The listing builds one solid part. Answer for the finished solid, in the listing's coordinates (mm). A direction names the side the tool comes from. Coordinates: 2 decimals unless noted, no trailing zeros. Loops run counter-clockwise (first coordinate to the right, second up) from the corner with the lowest first, then second, coordinate; pieces in that order, holes last. Notation, with made-up numbers: M 10,-7.5 L 67,-7.5 A14 cw 67,-3.5 Z; hole C 14.25,18 d1. An arc over 180 degrees is marked long. Answer as a JSON object with one key per item and string values. Group by question number.
1. For faces 1 (the face through (5.24, 3.65, -33.55)), 2 (the face through (-14.4, -1.7, 60.5)), 3 (the face through (-21, 9, -21)), determine the directions among +Z, -Z, +X, -X, +Y, -Y from which every point of the face is accessible in a straight line to the end or side of a thin tool.
2. Straight lines are drawn through the part: L1, parallel to Y at x = 24.5, z = -32.25; L2, parallel to Z at x = 25, y = -3; L3, parallel to Y at x = -28, z = 32. For each, find the intervals that lie inside material, in ascending order.
3. Given pin 1 (2 mm diameter, centred on x = 2, y = 1, fed in from -Z); pin 2 (2.5 mm diameter, centred on x = 24.5, y = 13.5, fed in from +Z); pin 3 (1 mm diameter, centred on x = -20.5, z = -25, fed in from +Y); pin 4 (8 mm diameter, centred on x = -1, y = 4.5, fed in from +Z), each flat-ended and moving along its own axis, determine where each tip first touches the part or whether it passes through.
4. A cutting plane is placed at B-B on x = -23.5. Give the vertices of the cut face in (y, z), and give its area (3 significant figures).
5. Determine the mould class of faces 4 (the face through (32.17, 9.19, 56.11)), 5 (the face through (29.076, 6.007, 58.084)), 6 (the face through (-22.434, -0.308, 48.794)) for opening direction Y: released by +Y, released by -Y, zero draft, split by the parting line, or undercut.
6. A cutting plane is placed at A-A on z = 32.5. Give the vertices of the cut face in (x, y), and give its area (3 significant figures).
7. A cutting plane is placed at D-D on z = -19. Give the vertices of the cut face in (x, y), and give its area (3 significant figures).
8. A cutting plane is placed at C-C on x = -3.5. Give the vertices of the cut face in (y, z), and give its area (3 significant figures).
from build123d import *

# Parameters (mm, degrees)
F0_W      = 2
F0_H      = 9
F0_W_2    = 24
F1_DEPTH  = 22
F3_R      = 20
F4_DEPTH  = 12
F5_R      = 5
F5_R_2    = 3.05
F6_DEPTH  = 50
F7_R      = 2
F8_DEPTH  = 9.001
F9_R      = 11
F10_DEPTH = 2
F11_R     = 1.5
F12_DEPTH = 20
F13_R     = 6
F14_DEPTH = 25
F15_DEPTH = 9


with BuildPart() as f1:
    # F0 (on Front) → F1 (new body, symmetric)
    with BuildSketch(Plane.XZ):
        with BuildLine():
            Line((-16, 51.5), (-16, 60.5))
            ThreePointArc((-16, 60.5), (-28.7279220614, 55.2279220614), (-34, 42.5))
            Line((-34, 42.5), (-34, -30))
            ThreePointArc((-34, -30), (-31.3639610307, -36.3639610307), (-25, -39))
            Line((-25, -39), (-25, -30))
            Line((-25, -30), (-25, 0))
            Line((-25, 0), (-25, 42.5))
            ThreePointArc((-25, 42.5), (-22.3639610307, 48.8639610307), (-16, 51.5))
        make_face()
        with Locations((-15, 56)):
            Rectangle(F0_W, F0_H)
        with Locations((-2, 56)):
            Rectangle(F0_W_2, F0_H)
        Polygon((-25, -30), (-25, -39), (29, -39), (29, -30), (-11.5, -30), align=None)
    extrude(amount=F1_DEPTH, both=True)

    # F0 (on Front) → F2 (revolve)
    with BuildSketch(Plane.XZ):
        Polygon((34, 64), (10, 64), (10, 60.5), (10, 51.5), (10, 48), (34, 48), align=None)
    revolve(axis=Axis((10, 0, 55.4929765165), (0, 0, -1)))

    # F3 (on face) → F4 (cut)
    with BuildSketch(Plane.XY.offset(64)):
        with Locations((10, 0)):
            Circle(F3_R)
    extrude(amount=-F4_DEPTH, mode=Mode.SUBTRACT)

    # F5 (on face) → F6 (cut)
    with BuildSketch(Plane.XY.offset(52)):
        with Locations((10, 0)):
            Circle(F5_R)
        with Locations((20, 0)):
            Circle(F5_R_2)
    extrude(amount=-F6_DEPTH, mode=Mode.SUBTRACT)

    # F7 (on face) → F8 (cut, through all)
    with BuildSketch(Plane.YZ.offset(-25)):
        with Locations((14, -22.5)):
            Circle(F7_R)
        with Locations((14, 32.5)):
            Circle(F7_R)
        with Locations((0, 32.5)):
            Circle(F7_R)
        with Locations((-14, -22.5)):
            Circle(F7_R)
        with Locations((-14, 32.5)):
            Circle(F7_R)
    extrude(amount=-F8_DEPTH, mode=Mode.SUBTRACT)

    # F9 (on face) → F10 (cut)
    with BuildSketch(Plane(origin=(0, 0, -39), x_dir=(1, 0, 0), z_dir=(0, 0, -1))):
        with Locations((10, 0)):
            Circle(F9_R)
    extrude(amount=-F10_DEPTH, mode=Mode.SUBTRACT)

    # F11 (on face) → F12 (cut)
    with BuildSketch(Plane(origin=(0, 0, -39), x_dir=(1, 0, 0), z_dir=(0, 0, -1))):
        with Locations((-3.5, -13.5)):
            Circle(F11_R)
        with Locations((-3.5, 14.5)):
            Circle(F11_R)
        with Locations((24.5, -13.5)):
            Circle(F11_R)
        with Locations((24.5, 14.5)):
            Circle(F11_R)
        with Locations((52.5, -13.5)):
            Circle(F11_R)
        with Locations((52.5, 14.5)):
            Circle(F11_R)
    extrude(amount=-F12_DEPTH, mode=Mode.SUBTRACT)

    # F13 (on face) → F14 (cut)
    with BuildSketch(Plane(origin=(0, 0, -39), x_dir=(1, 0, 0), z_dir=(0, 0, -1))):
        with Locations((10, 0)):
            Circle(F13_R)
    extrude(amount=-F14_DEPTH, mode=Mode.SUBTRACT)

    # F0 (on Front) → F15 (join, symmetric)
    with BuildSketch(Plane.XZ):
        Polygon((-11.5, -30), (-25, 0), (-25, -30), align=None)
    extrude(amount=F15_DEPTH, both=True)


solid = f1.part
From the geometry:
{
 "1": {"face 1": "-Z", "face 2": "+Z, -X", "face 3": "+X, +Y"},
 "2": {"L1": "y = -22 to -16, -13 to 12, 15 to 22", "L2": "z = -39 to -30, 48 to 52", "L3": "y = -22 to -15.94, -12.06 to -1.94, 1.94 to 12.06, 15.94 to 22"},
 "3": {"pin 1": "stops at z = -37", "pin 2": "stops at z = 64", "pin 3": "stops at y = 9", "pin 4": "stops at z = 52"},
 "4": {"outline": "M -22,-39 L 22,-39 L 22,-30 L 9,-30 L 9,-3.33 L -9,-3.33 L -9,-30 L -22,-30 Z; M -22,47.47 L 22,47.47 L 22,58.86 L -22,58.86 Z", "area": "1,380 mm²"},
 "5": {"face 4": "split by the parting line", "face 5": "undercut", "face 6": "zero draft"},
 "6": {"outline": "M -34,-22 L -25,-22 L -25,-16 L -34,-16 Z; M -34,-12 L -25,-12 L -25,-2 L -34,-2 Z; M -34,2 L -25,2 L -25,12 L -34,12 Z; M -34,16 L -25,16 L -25,22 L -34,22 Z", "area": "288 mm²"},
 "7": {"outline": "M -34,-22 L -25,-22 L -25,-9 L -16.45,-9 L -16.45,9 L -25,9 L -25,22 L -34,22 Z", "area": "550 mm²"},
 "8": {"outline": "M -22,-39 L -16,-39 L -16,-30 L -22,-30 Z; M -22,51.5 L -19.84,51.5 L -19.84,48 L 19.84,48 L 19.84,51.5 L 22,51.5 L 22,60.5 L 19.84,60.5 L 19.84,64 L 14.76,64 L 14.76,52 L -14.76,52 L -14.76,64 L -19.84,64 L -19.84,60.5 L -22,60.5 Z; M -13,-39 L 12,-39 L 12,-30 L -13,-30 Z; M 15,-39 L 22,-39 L 22,-30 L 15,-30 Z", "area": "662 mm²"}
}
